Verification items for the finished model (mm, model axes). A direction names the side the tool comes from. Coordinates: 2 decimals unless noted, no trailing zeros. Order: outer loops, then holes, each group sorted by start corner. A loop starts at its lowest first (then second) coordinate and runs counter-clockwise, first axis right, second up. Notation, with made-up numbers: (56.5, 55.25) - (73.5, 55.25) arc R33 ccw to (73.5, 85.25) - close; hole circle Ø3 at (64.25, -38.5). An arc over 180 degrees is marked (long way). Answer as CSV lines item,"result". Start each with the question number.
1. Section check A-A (y = 10.25). Count the separate pieces of the cut face and the enclosed holes in it, and give its area (3 significant figures).
2. Material ranges on L1, parallel to X at y = 9.25, z = -70.5; L2, parallel to Z at x = 93.5, y = 4; L3, parallel to Z at x = 113.5, y = 5.5, recorded low to high. Write a range as [from, to].
3. Section check C-C (z = -44.5). Record the cut outline in (x, y), and give its area (3 significant figures).
4. Section check B-B (x = 27.5). Record the cut outline in (y, z).
5. Set-up check for faces 4 (the cylindrical face through (49.6, 7.9, -68.7)), 5 (the flat face through (77, 13, -70)): record each of +Z, -Z, +X, -X, +Y, -Y from which the full face is reachable in a straight line by a thin tool's end or side.
6. Section check D-D (x = 66.5). Record the cut outline in (y, z), and give its area (3 significant figures).
7. Go/stop test with flat-tipped pins: pin 1 (5 mm diameter, centred on x = 62, y = 10.5, fed in from +Z); pin 2 (2.5 mm diameter, centred on x = 52, z = -70.5, fed in from +Y); pin 3 (1 mm diameter, centred on y = 4, z = -23.5, fed in from +X). Record where each tip stops, or that it passes through.
8. Mould release check, pull along Z, two halves, no side actions. Record for faces 1 (the flat face through (60, 1, -78)), 2 (the flat face through (53, 13, -73)), 3 (the cylindrical face through (108.04, 7.93, -68.45)): pulls with the +Z half, pulls with the -Z half, needs draft (parallel to the pull), parting line crosses it, or undercut.
from build123d import *

# Parameters (mm, degrees)
SKETCH6_W            = 121
SKETCH6_H            = 78
BOSS_EXTRUDE9_DEPTH  = 3
SKETCH14_W           = 117
SKETCH14_H           = 74
SKETCH14_W_2         = 113
SKETCH14_H_2         = 70
BOSS_EXTRUDE11_DEPTH = 2
SKETCH16_R           = 3
SKETCH16_R_2         = 2.1
BOSS_EXTRUDE12_DEPTH = 10
SKETCH17_R           = 3
SKETCH17_R_2         = 2.1
BOSS_EXTRUDE13_DEPTH = 10
SKETCH18_R           = 3
SKETCH18_R_2         = 2.1
BOSS_EXTRUDE14_DEPTH = 10
SKETCH19_R           = 3
SKETCH19_R_2         = 2.1
BOSS_EXTRUDE15_DEPTH = 10
SKETCH20_R           = 3
SKETCH20_R_2         = 2.1
BOSS_EXTRUDE16_DEPTH = 10
SKETCH21_R           = 3
SKETCH21_R_2         = 2.1
BOSS_EXTRUDE17_DEPTH = 10
CUT_EXTRUDE2_DEPTH   = 1


with BuildPart() as part:
    # Sketch6 → Boss-Extrude9 (new body)
    with BuildSketch(Plane(origin=(0, 0, 0), x_dir=(1, 0, 0), z_dir=(0, 1, 0))):
        with Locations((60.5, 39)):
            Rectangle(SKETCH6_W, SKETCH6_H)
    extrude(amount=BOSS_EXTRUDE9_DEPTH)

    # Sketch14 → Boss-Extrude11 (add)
    with BuildSketch(Plane(origin=(0, 3, 0), x_dir=(1, 0, 0), z_dir=(0, 1, 0))):
        with Locations((60.5, 39)):
            Rectangle(SKETCH14_W, SKETCH14_H)
        with Locations((60.5, 39)):
            Rectangle(SKETCH14_W_2, SKETCH14_H_2, mode=Mode.SUBTRACT)
    extrude(amount=BOSS_EXTRUDE11_DEPTH)

    # Sketch16 → Boss-Extrude12 (add)
    with BuildSketch(Plane(origin=(0, 3, 0), x_dir=(1, 0, 0), z_dir=(0, 1, 0))):
        with Locations((52, 70.5)):
            Circle(SKETCH16_R)
        with Locations((52, 70.5)):
            Circle(SKETCH16_R_2, mode=Mode.SUBTRACT)
    extrude(amount=BOSS_EXTRUDE12_DEPTH)

    # Sketch17 → Boss-Extrude13 (add)
    with BuildSketch(Plane(origin=(0, 3, 0), x_dir=(1, 0, 0), z_dir=(0, 1, 0))):
        with Locations((108.5, 70.5)):
            Circle(SKETCH17_R)
        with Locations((108.5, 70.5)):
            Circle(SKETCH17_R_2, mode=Mode.SUBTRACT)
    extrude(amount=BOSS_EXTRUDE13_DEPTH)

    # Sketch18 → Boss-Extrude14 (add)
    with BuildSketch(Plane(origin=(0, 3, 0), x_dir=(1, 0, 0), z_dir=(0, 1, 0))):
        with Locations((79.5, 70.5)):
            Circle(SKETCH18_R)
        with Locations((79.5, 70.5)):
            Circle(SKETCH18_R_2, mode=Mode.SUBTRACT)
    extrude(amount=BOSS_EXTRUDE14_DEPTH)

    # Sketch19 → Boss-Extrude15 (add)
    with BuildSketch(Plane(origin=(0, 3, 0), x_dir=(1, 0, 0), z_dir=(0, 1, 0))):
        with Locations((10, 20.2)):
            Circle(SKETCH19_R)
        with Locations((10, 20.2)):
            Circle(SKETCH19_R_2, mode=Mode.SUBTRACT)
    extrude(amount=BOSS_EXTRUDE15_DEPTH)

    # Sketch20 → Boss-Extrude16 (add)
    with BuildSketch(Plane(origin=(0, 3, 0), x_dir=(1, 0, 0), z_dir=(0, 1, 0))):
        with Locations((113.5, 18.2)):
            Circle(SKETCH20_R)
        with Locations((113.5, 18.2)):
            Circle(SKETCH20_R_2, mode=Mode.SUBTRACT)
    extrude(amount=BOSS_EXTRUDE16_DEPTH)

    # Sketch21 → Boss-Extrude17 (add)
    with BuildSketch(Plane(origin=(0, 3, 0), x_dir=(1, 0, 0), z_dir=(0, 1, 0))):
        with Locations((66.5, 20)):
            Circle(SKETCH21_R)
        with Locations((66.5, 20)):
            Circle(SKETCH21_R_2, mode=Mode.SUBTRACT)
    extrude(amount=BOSS_EXTRUDE17_DEPTH)

    # Sketch22 → Cut-Extrude2 (cut)
    with BuildSketch(Plane(origin=(0, 0, 0), x_dir=(-1, 0, 0), z_dir=(0, -1, 0))):
        with BuildLine():
            Line((-59.348084392, 41.348070521), (-59.348084392, 41.022429495))
            Line((-59.348084392, 41.022429495), (-60.428042325, 41.022429495))
            Line((-60.428042325, 41.022429495), (-60.599131067, 40.187338349))
            add(Edge.make_bspline(
                [(-60.599131067, 40.187338349), (-60.565516095, 40.196618667), (-60.500392404, 40.214597816), (-60.404271673, 40.234560193), (-60.313020174, 40.246593846), (-60.253806088, 40.248236963), (-60.225152702, 40.249032059)],
                knots=[0, 0, 0, 0, 0.000104595, 0.000202637, 0.000294305, 0.000380252, 0.000380252, 0.000380252, 0.000380252], degree=3))
            add(Edge.make_bspline(
                [(-60.225152702, 40.249032059), (-60.189698166, 40.248264675), (-60.119985692, 40.246755805), (-60.017987504, 40.232267056), (-59.920621236, 40.209461562), (-59.828090515, 40.177602232), (-59.740224158, 40.136862688), (-59.657830585, 40.085972028), (-59.579673049, 40.026523934), (-59.507153696, 39.958175245), (-59.441363788, 39.882953493), (-59.383518926, 39.802074567), (-59.334385719, 39.716324473), (-59.294869892, 39.624883921), (-59.263315531, 39.528763832), (-59.242313364, 39.426952846), (-59.228328207, 39.320410623), (-59.226765757, 39.247562906), (-59.225969008, 39.210415273)],
                knots=[0, 0, 0, 0, 0.000106308, 0.000209029, 0.000308378, 0.000405929, 0.000502102, 0.000598312, 0.00069588, 0.000796219, 0.000896736, 0.000995218, 0.001094066, 0.001192613, 0.001293582, 0.001396995, 0.001504047, 0.001615439, 0.001615439, 0.001615439, 0.001615439], degree=3))
            add(Edge.make_bspline(
                [(-59.225969008, 39.210415273), (-59.226572326, 39.184541544), (-59.227770809, 39.133143748), (-59.233865528, 39.056812938), (-59.24560007, 38.982098082), (-59.261355077, 38.908989269), (-59.281804271, 38.83762491), (-59.306559341, 38.767800738), (-59.336854309, 38.699951345), (-59.370084199, 38.633434737), (-59.407500647, 38.569754662), (-59.449028293, 38.510201653), (-59.492902703, 38.453882341), (-59.540111674, 38.40140074), (-59.591094005, 38.353101717), (-59.645232261, 38.308698633), (-59.702094442, 38.267440569), (-59.762560269, 38.231002278), (-59.825282378, 38.197471596), (-59.891166547, 38.169963816), (-59.958713039, 38.145370694), (-60.028894034, 38.125767765), (-60.101550564, 38.110407519), (-60.176802396, 38.099974831), (-60.254254861, 38.092376206), (-60.306755765, 38.091900539), (-60.333275698, 38.091660265)],
                knots=[0, 0, 0, 0, 7.7636e-05, 0.000154223, 0.000229512, 0.000304362, 0.000378447, 0.000452077, 0.000526407, 0.000601214, 0.00067506, 0.000747747, 0.00081887, 0.000889121, 0.000959302, 0.001029336, 0.001099058, 0.00116985, 0.001240974, 0.00131221, 0.00138383, 0.001456517, 0.001530612, 0.001606437, 0.001684346, 0.001763871, 0.001763871, 0.001763871, 0.001763871], degree=3))
            add(Edge.make_bspline(
                [(-60.333275698, 38.091660265), (-60.364911562, 38.092286953), (-60.427151387, 38.093519889), (-60.518337902, 38.106418087), (-60.606071865, 38.124891068), (-60.689647029, 38.152682541), (-60.769812389, 38.187505301), (-60.845488712, 38.2315164), (-60.918609666, 38.281390301), (-60.986202728, 38.34024605), (-61.048937202, 38.404576704), (-61.105095249, 38.474388279), (-61.15510928, 38.548528558), (-61.198178379, 38.627357598), (-61.23491587, 38.710668266), (-61.263776609, 38.798772702), (-61.287070545, 38.891210563), (-61.296925219, 38.954849819), (-61.301930546, 38.987173085)],
                knots=[0, 0, 0, 0, 9.4843e-05, 0.000186593, 0.000275792, 0.000363484, 0.000450342, 0.000537514, 0.000625728, 0.000715478, 0.000805885, 0.000894984, 0.00098389, 0.001073836, 0.001164117, 0.001256635, 0.001351658, 0.001449737, 0.001449737, 0.001449737, 0.001449737], degree=3))
            Line((-61.301930546, 38.987173085), (-61.016994649, 38.987173085))
            add(Edge.make_bspline(
                [(-61.016994649, 38.987173085), (-61.009983743, 38.956895875), (-60.996508393, 38.898701395), (-60.966930321, 38.816939392), (-60.930766277, 38.744078382), (-60.887763761, 38.679154546), (-60.836464805, 38.62254067), (-60.777927394, 38.57208805), (-60.712297674, 38.526572039), (-60.63936953, 38.488632815), (-60.562431951, 38.45627616), (-60.48190741, 38.43472998), (-60.399988467, 38.419579884), (-60.34458166, 38.418063358), (-60.31673924, 38.41730129)],
                knots=[0, 0, 0, 0, 9.3172e-05, 0.000179081, 0.000260145, 0.000336703, 0.000411917, 0.000488562, 0.000568128, 0.000650923, 0.00073478, 0.000817953, 0.000900557, 0.000983994, 0.000983994, 0.000983994, 0.000983994], degree=3))
            add(Edge.make_bspline(
                [(-60.31673924, 38.41730129), (-60.289562651, 38.418045853), (-60.236051725, 38.419511903), (-60.157301396, 38.430795864), (-60.081271146, 38.448174518), (-60.008711186, 38.474182172), (-59.93835179, 38.50579131), (-59.871972727, 38.546354271), (-59.807653688, 38.59303586), (-59.747393881, 38.646517945), (-59.692203809, 38.70545474), (-59.643439328, 38.768480661), (-59.602820271, 38.835715229), (-59.568590044, 38.905994446), (-59.542597408, 38.980088566), (-59.524054518, 39.057650346), (-59.513166029, 39.138871364), (-59.511668173, 39.194269952), (-59.510904905, 39.222499607)],
                knots=[0, 0, 0, 0, 8.15e-05, 0.000160473, 0.000238226, 0.000315066, 0.000391338, 0.000469218, 0.000547964, 0.000629516, 0.000710512, 0.000789892, 0.000868102, 0.000945761, 0.001024012, 0.00110315, 0.001184644, 0.001269321, 0.001269321, 0.001269321, 0.001269321], degree=3))
            add(Edge.make_bspline(
                [(-59.510904905, 39.222499607), (-59.51150224, 39.247968325), (-59.512671438, 39.297819716), (-59.52222417, 39.370753282), (-59.53884028, 39.439762399), (-59.561903372, 39.505180311), (-59.591185496, 39.567068719), (-59.626968937, 39.625491495), (-59.669925234, 39.679678615), (-59.718994304, 39.729655432), (-59.772749813, 39.775778997), (-59.832116636, 39.815098275), (-59.895852427, 39.848176258), (-59.963189278, 39.876722228), (-60.035728864, 39.897224333), (-60.112034667, 39.912616629), (-60.19293068, 39.921520565), (-60.248239805, 39.922755992), (-60.276670129, 39.923391034)],
                knots=[0, 0, 0, 0, 7.6388e-05, 0.000149519, 0.000220172, 0.000288967, 0.000357247, 0.000425206, 0.000494043, 0.000564207, 0.000635056, 0.000706145, 0.000777268, 0.000850264, 0.000925136, 0.001002969, 0.001083601, 0.001168886, 0.001168886, 0.001168886, 0.001168886], degree=3))
            add(Edge.make_bspline(
                [(-60.276670129, 39.923391034), (-60.301279943, 39.922864355), (-60.352092966, 39.921776896), (-60.430037244, 39.913770002), (-60.511944736, 39.900852928), (-60.597501457, 39.883085404), (-60.686964346, 39.859834355), (-60.78014461, 39.831971916), (-60.877238166, 39.798659817), (-60.942659245, 39.773502737), (-60.97628952, 39.760570521)],
                knots=[0, 0, 0, 0, 7.3822e-05, 0.000152423, 0.000234822, 0.000322511, 0.00041445, 0.000512043, 0.000614219, 0.000722306, 0.000722306, 0.000722306, 0.000722306], degree=3))
            Line((-60.97628952, 39.760570521), (-60.650648495, 41.348070521))
            Line((-60.650648495, 41.348070521), (-59.348084392, 41.348070521))
        make_face()
        Polygon((-57.167179945, 41.429480777), (-57.109302341, 41.429480777), (-57.109302341, 39.231403854), (-56.742956187, 39.231403854), (-56.742956187, 38.905762829), (-57.109302341, 38.905762829), (-57.109302341, 38.173070521), (-57.394238238, 38.173070521), (-57.394238238, 38.905762829), (-58.900327982, 38.905762829), align=None)
        Polygon((-57.394238238, 39.231403854), (-57.394238238, 40.610290072), (-58.340632469, 39.231403854), align=None, mode=Mode.SUBTRACT)
    extrude(amount=-CUT_EXTRUDE2_DEPTH, mode=Mode.SUBTRACT)


solid = part.part
Evaluation:
1,separate pieces,"6"
1,enclosed holes,"6"
1,area,"86.5 mm²"
2,L1,"x = [49, 49.9], [54.1, 55], [76.5, 77.4], [81.6, 82.5], [105.5, 106.4], [110.6, 111.5]"
2,L2,"z = [-76, -74], [-4, -2]"
2,L3,"z = [-21.2, -20.3], [-16.1, -15.2]"
3,outline,"(0, 0) - (121, 0) - (121, 3) - (119, 3) - (119, 5) - (117, 5) - (117, 3) - (4, 3) - (4, 5) - (2, 5) - (2, 3) - (0, 3) - close"
3,area,"371 mm²"
4,outline,"(0, -78) - (3, -78) - (3, -76) - (5, -76) - (5, -74) - (3, -74) - (3, -4) - (5, -4) - (5, -2) - (3, -2) - (3, 0) - (0, 0) - close"
5,face 4,"+Y"
5,face 5,"+Z, -Z, +X, -X, +Y"
6,outline,"(0, -78) - (3, -78) - (3, -76) - (5, -76) - (5, -74) - (3, -74) - (3, -23) - (13, -23) - (13, -22.1) - (3, -22.1) - (3, -17.9) - (13, -17.9) - (13, -17) - (3, -17) - (3, -4) - (5, -4) - (5, -2) - (3, -2) - (3, 0) - (0, 0) - close"
6,area,"260 mm²"
7,pin 1,"stops at z = -17.76"
7,pin 2,"stops at y = 3"
7,pin 3,"stops at x = 119"
8,face 1,"pulls with the -Z half"
8,face 2,"needs draft"
8,face 3,"undercut"
